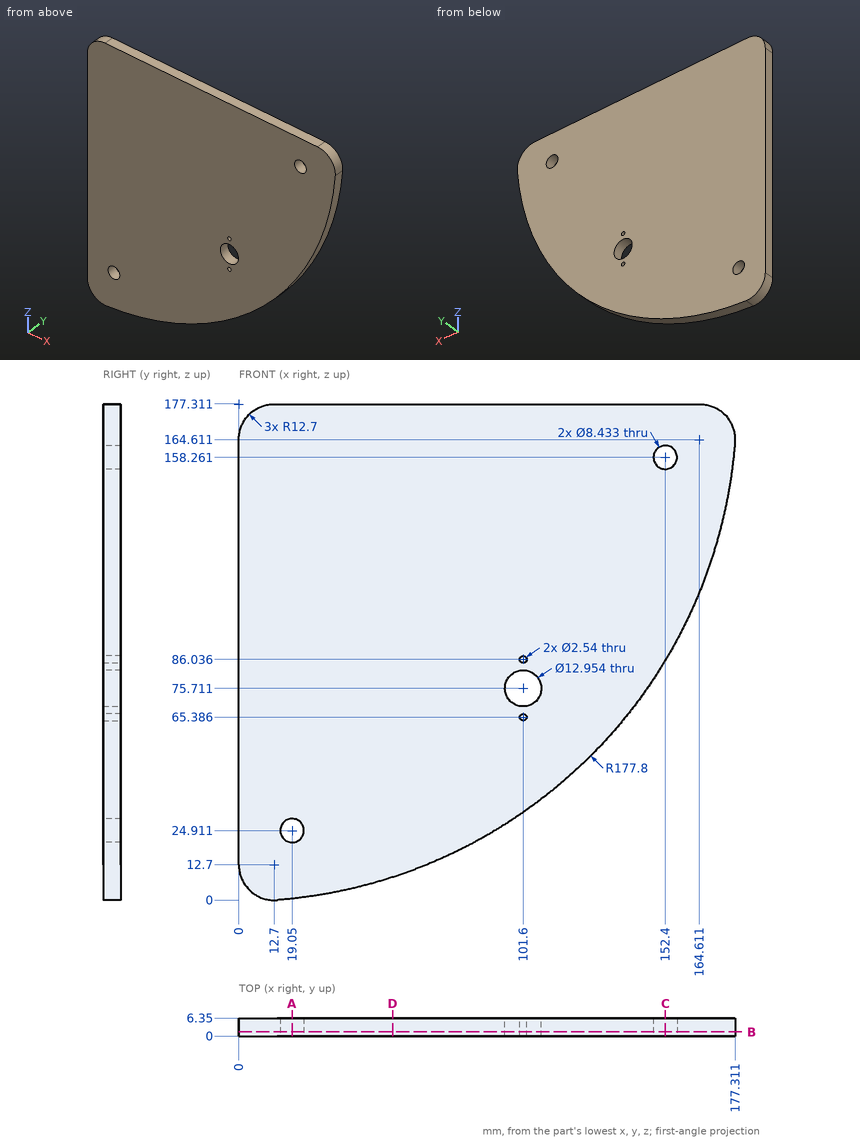
Could you check a few things on this drawing? It's one solid part, dimensions in mm from its lowest x, y, z. Round coordinates to 2 decimals unless told otherwise and drop trailing zeros. Order: outer loops, then holes, each group sorted by start corner. A loop starts at its lowest first (then second) coordinate and runs counter-clockwise, first axis right, second up. Notation, with made-up numbers: M 1,45.5 L 15,45.5 A21 cw 15,68.5 Z; hole C 39.5,27.25 d9. An arc over 180 degrees is marked long. One line per question, with ' | ' between items. Start each with the question number.
(1) Suppose I cut it at A-A on x = 19.05. List the corners of the cut face in (y, z) for me.
(2) Suppose I cut it at B-B on y = 1.5. List the corners of the cut face in (x, z) for me, then the cut area to 3 significant figures.
(3) Suppose I cut it at C-C on x = 152.4. List the corners of the cut face in (y, z) for me, then the cut area to 3 significant figures.
(4) Please list where these lines run through material, in increasing order: line 1 along Z through (x, y) = (69.5, 6); line 2 along X through (y, z) = (5.75, 28) (1 decimal); line 3 along X through (y, z) = (0.5, 30.5) (1 decimal).
(5) Suppose I cut it at D-D on x = 55. List the corners of the cut face in (y, z) for me, then the cut area to 3 significant figures.
(6) For P1, Ø1.5, axis at x = 101.6, z = 86.04, coming from the -Y side; P2, Ø3, axis at x = 39.5, y = 1.5, coming from the -Z side; P3, Ø3, axis at y = 3, z = 115.5, coming from the +X side; P4, Ø9.5, axis at x = 19.05, z = 24.91, coming from the +Y side, each with a flat end and sliding along its axis, tell me the tip position at first contact or that it passes through.
Geometry results:
1) outline: M 0,0.53 L 6.35,0.53 L 6.35,20.69 L 0,20.69 Z; M 0,29.13 L 6.35,29.13 L 6.35,177.31 L 0,177.31 Z
2) outline: M 0,12.7 A12.7 ccw 13.68,0.04 A177.8 ccw 177.27,163.63 A12.7 ccw 164.61,177.31 L 12.7,177.31 A12.7 ccw 0,164.61 Z; hole C 19.05,24.91 d8.43; hole C 101.6,75.71 d12.95; hole C 101.6,65.39 d2.54; hole C 101.6,86.04 d2.54; hole C 152.4,158.26 d8.43 | area: 24,500 mm²
3) outline: M 0,85.73 L 6.35,85.73 L 6.35,154.04 L 0,154.04 Z; M 0,162.48 L 6.35,162.48 L 6.35,177.31 L 0,177.31 Z | area: 528 mm²
4) line 1: 13.66 to 177.31 | line 2: 0 to 16.2, 21.9 to 96.5 | line 3: 0 to 100.3
5) outline: M 0,8.23 L 6.35,8.23 L 6.35,177.31 L 0,177.31 Z | area: 1,070 mm²
6) P1: through | P2: z = 3.62 | P3: x = 167.26 | P4: y = 6.35
